from build123d import *

# Parameters (mm, degrees)
SKETCH_1_W          = 29
SKETCH_1_H          = 28
EXTRUDE_3_DEPTH     = 30
SKETCH_2_W          = 19
SKETCH_2_H          = 6
EXTRUDE_4_DEPTH     = 35
SKETCH_3_R          = 2
CUT_EXTRUDE_3_DEPTH = 48.108916353
SKETCH_4_W          = 25.2
SKETCH_4_H          = 24.2
CUT_EXTRUDE_4_DEPTH = 18
CUT_EXTRUDE_START   = -18
SKETCH_4_3_R        = 5.1
CUT_EXTRUDE_5_DEPTH = 10
FILLET_1_R          = 5
FILLET_2_R          = 9.5


with BuildPart() as part:
    # 草图1 → 凸台-拉伸3 (new body)
    with BuildSketch(Plane(origin=(0, 0, 0), x_dir=(1, 0, 0), z_dir=(0, 1, 0))):
        Rectangle(SKETCH_1_W, SKETCH_1_H)
    extrude(amount=EXTRUDE_3_DEPTH)

    # 草图2 → 凸台-拉伸4 (add)
    with BuildSketch(Plane.XZ):
        with Locations((0, -11)):
            Rectangle(SKETCH_2_W, SKETCH_2_H)
        with Locations((0, 11)):
            Rectangle(SKETCH_2_W, SKETCH_2_H)
    extrude(amount=EXTRUDE_4_DEPTH)

    # 草图3 → 切除-拉伸3 (cut, through all)
    with BuildSketch(Plane(origin=(0, 0, -14), x_dir=(-1, 0, 0), z_dir=(0, 0, -1))):
        with Locations((0, -25)):
            Circle(SKETCH_3_R)
    extrude(amount=-CUT_EXTRUDE_3_DEPTH, mode=Mode.SUBTRACT)

    # 草图4 → 切除-拉伸4 (cut)
    with BuildSketch(Plane(origin=(0, 30, 0), x_dir=(1, 0, 0), z_dir=(0, 1, 0))):
        Rectangle(SKETCH_4_W, SKETCH_4_H)
    extrude(amount=-CUT_EXTRUDE_4_DEPTH, mode=Mode.SUBTRACT)

    # 草图4<3> → 切除-拉伸5 (cut)
    with BuildSketch(Plane(origin=(0, 30, 0), x_dir=(1, 0, 0), z_dir=(0, 1, 0)).offset(CUT_EXTRUDE_START)):
        with Locations(Location((0, 0, 0), (0, 0, 270))):
            Circle(SKETCH_4_3_R)
    extrude(amount=-CUT_EXTRUDE_5_DEPTH, mode=Mode.SUBTRACT)

    # 圆角1
    fillet_1_edges = [part.edges().sort_by_distance(p)[0] for p in [
        (-14.5, 0, 0),
        (14.5, 0, 0),
    ]]
    fillet(fillet_1_edges, radius=FILLET_1_R)

    # 圆角2
    fillet_2_edges = [part.edges().sort_by_distance(p)[0] for p in [
        (9.5, -35, -11),
        (-9.5, -35, -11),
        (9.5, -35, 11),
        (-9.5, -35, 11),
    ]]
    fillet(fillet_2_edges, radius=FILLET_2_R - 0.0001)  # a hair under: the kernel refuses the full size


solid = part.part
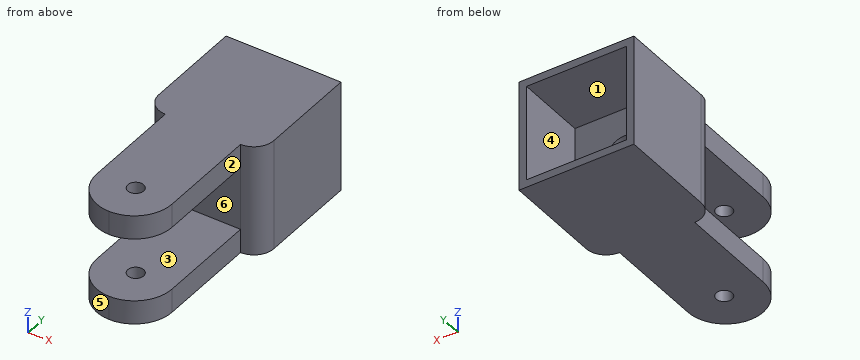
Design review of the part built by this model. Coordinates are the model's own, in mm. Face numbers are marked on the shaded views. A direction names the side the tool comes from. Round coordinates to 2 decimals unless told otherwise and drop trailing zeros. Write each loop counter-clockwise with the first axis right and the second up, starting at its lowest first coordinate (ties: lowest second). Pieces come first, ordered by that corner, then holes.
Item 1: For the marked faces 1, 2 and 3, list the 3-axis set-ups (+Z, -Z, +X, -X, +Y, -Y) from which the entire face can be reached by the end or side of a thin tool; tool diameter is ignored.
Item 2: Consider section A-A on y = -3.5. Give the boundary of the cut face in (x, z), and give its area (3 significant figures).
Item 3: Consider section D-D on y = 18. Give the boundary of the cut face in (x, z), and give its area (3 significant figures).
Item 4: For pin 1 Ø16.5 at (x, z) = (0, 0) entering from -Y; pin 2 Ø1.5 at (x, z) = (-9, 1) entering from +Y; pin 3 Ø5 at (x, z) = (9, 10) entering from -Y; pin 4 Ø3 at (y, z) = (-12.5, -11) entering from +X, all flat-tipped, find the tip position at first contact; note any pin that passes through.
Item 5: Consider section C-C on x = 1.25. Give the boundary of the cut face in (y, z).
Item 6: Draft analysis for pull direction X (two halves, no side actions). For the marked faces 4, 5 and 6, state which applies: released by +X, released by -X, zero draft, split by the parting line, or undercut.
Item 7: Wall thickness on L1, parallel to X at y = 6.5, z = 0; L2, parallel to Y at x = 0, z = -10.3; L3, parallel to X at y = 17.5, z = 3.5: over which ranges is each line inside the solid? List them lowest first.
Check values:
1. face 1: +Y
1. face 2: +Z, -Z, +X, -Y
1. face 3: +X, -X, -Y
2. outline: (-9.5, -14) - (9.5, -14) - (9.5, -8) - (-9.5, -8) - close; (-9.5, 8) - (9.5, 8) - (9.5, 14) - (-9.5, 14) - close
2. area: 228 mm2
3. outline: (-14.5, -14) - (14.5, -14) - (14.5, 14) - (-14.5, 14) - close; hole (-12.6, -12.1) - (12.6, -12.1) - (12.6, 12.1) - (-12.6, 12.1) - close
3. area: 202 mm2
4. pin 1: stops at y = -35
4. pin 2: stops at y = 12
4. pin 3: stops at y = -32.43
4. pin 4: stops at x = 9.5
5. outline: (-34.92, -14) - (-26.56, -14) - (-26.56, -8) - (-34.92, -8) - close; (-34.92, 8) - (-26.56, 8) - (-26.56, 14) - (-34.92, 14) - close; (-23.44, -14) - (30, -14) - (30, -12.1) - (12, -12.1) - (12, -4.94) - (2, -4.94) - (2, 4.94) - (12, 4.94) - (12, 12.1) - (30, 12.1) - (30, 14) - (-23.44, 14) - (-23.44, 8) - (0, 8) - (0, -8) - (-23.44, -8) - close
6. face 4: undercut
6. face 5: released by -X
6. face 6: zero draft
7. L1: x = -14.5 to -5.1, 5.1 to 14.5
7. L2: y = -35 to -27, -23 to 12
7. L3: x = -14.5 to -12.6, 12.6 to 14.5
